Part model, mm, in its own coordinate system. Give positions to 0.01 mm unless a question says otherwise; leave off trailing zeros. Write each loop counter-clockwise with the first axis right and the second up, starting at its lowest first coordinate (ties: lowest second). Pieces come first, ordered by that corner, then holes. Notation, with made-up numbers: M 85,79 L 100,79 A23 ccw 100,87 Z; hole C 49,-5.75 d10. An arc over 180 degrees is marked long. Answer as CSV lines item,"result". Start each with the question number.
Item 1: Wall check: L1, parallel to X at y = -1.3, z = 46.5; L2, parallel to Y at x = -0.2, z = 2; L3, parallel to Z at x = 1.5, y = 2.25. Give the ranges that are in metal, low to high. Write a range as from..to.
Item 2: Pin check, flat tips, straight feed: pin 1 (1 mm diameter, centred on x = -2, z = -32, fed in from +Y); pin 2 (3 mm diameter, centred on x = -2, z = 5.5, fed in from +Y). Stop position of each tip, or through.
Item 3: Band-saw the part on A-A, the plane z = 34. List the corners of the cut face in (x, y).
from build123d import *

# Parameters (mm, degrees)
SKETCH_1_R      = 3
EXTRUDE_1_DEPTH = 60
CHAMFER_1_SIZE  = 0.3
CHAMFER_2_SIZE  = 0.3


with BuildPart() as part:
    # 草图1 → 凸台-拉伸1 (new, symmetric)
    with BuildSketch(Plane.XY):
        Circle(SKETCH_1_R)
    extrude(amount=EXTRUDE_1_DEPTH, both=True)

    # 倒角1
    chamfer_1_edges = [part.edges().sort_by_distance(p)[0] for p in [
        (-3, 0, 60),
    ]]
    chamfer(chamfer_1_edges, length=CHAMFER_1_SIZE)

    # 倒角2
    chamfer_2_edges = [part.edges().sort_by_distance(p)[0] for p in [
        (-3, 0, -60),
    ]]
    chamfer(chamfer_2_edges, length=CHAMFER_2_SIZE)


solid = part.part
Output:
1,L1,"-2.7..2.7"
1,L2,"-2.99..2.99"
1,L3,"-60..60"
2,pin 1,"y = 2.6"
2,pin 2,"y = 2.96"
3,outline,"C 0,0 d6"
